Geometry check sheet. Reference: the model listing, model coordinates, mm. A direction names the side the tool comes from. Round coordinates to 2 decimals unless told otherwise and drop trailing zeros. Loops run counter-clockwise (first coordinate to the right, second up) from the corner with the lowest first, then second, coordinate; pieces in that order, holes last. Notation, with made-up numbers: M -17,71 L -12,71 A24 ccw -12,89 Z; hole C 14.5,31 d7. An arc over 180 degrees is marked long. Answer in a Markdown table with one row per item. Add a question column.
```python
from build123d import *

# Parameters (mm, degrees)
BOX035_W               = 60
BOX035_H               = 3
BOX035_DEPTH           = 11
BOX034_W               = 200
BOX034_H               = 30
BOX034_DEPTH           = 20
BOX033_W               = 60
BOX033_H               = 3
BOX033_DEPTH           = 11
BOX025_W               = 3
BOX025_H               = 20
BOX025_DEPTH           = 11
BOX026_W               = 3
BOX026_H               = 20
BOX026_DEPTH           = 11
BOX024_W               = 30
BOX024_H               = 20
BOX024_DEPTH           = 11
BOX023_W               = 20
BOX023_H               = 20
BOX023_DEPTH           = 11
CUT010_PLACEMENT_ANGLE = 180
BOX032_W               = 30
BOX032_H               = 20
BOX032_DEPTH           = 11
BOX031_W               = 20
BOX031_H               = 20
BOX031_DEPTH           = 11
CUT013_PLACEMENT_ANGLE = 180
BOX030_W               = 30
BOX030_H               = 20
BOX030_DEPTH           = 11
BOX029_W               = 20
BOX029_H               = 20
BOX029_DEPTH           = 11
CUT012_PLACEMENT_ANGLE = 180
BOX022_W               = 30
BOX022_H               = 20
BOX022_DEPTH           = 11
BOX021_W               = 20
BOX021_H               = 20
BOX021_DEPTH           = 11
CHAMFER006_SIZE        = 4
BOX018_W               = 178
BOX018_H               = 104
BOX018_DEPTH           = 30
BOX019_W               = 181
BOX019_H               = 121
BOX019_DEPTH           = 5
BOX017_W               = 186
BOX017_H               = 127
BOX017_DEPTH           = 4
FILLET008_R            = 2
FILLET009_R            = 1


with BuildPart() as cube032:
    # Box035 → Box035 (new body)
    with BuildSketch(Plane(origin=(63, 0, 4), x_dir=(1, 0, 0), z_dir=(0, 0, 1))):
        with Locations((30, 1.5)):
            Rectangle(BOX035_W, BOX035_H)
    extrude(amount=BOX035_DEPTH)


with BuildPart() as cube031:
    # Box034 → Box034 (new body)
    with BuildSketch(Plane(origin=(-10, 73, -5), x_dir=(1, 0, 0), z_dir=(0, 0, 1))):
        with Locations((100, 15)):
            Rectangle(BOX034_W, BOX034_H)
    extrude(amount=BOX034_DEPTH)


with BuildPart() as cube030:
    # Box033 → Box033 (new body)
    with BuildSketch(Plane(origin=(63, 112, 4), x_dir=(1, 0, 0), z_dir=(0, 0, 1))):
        with Locations((30, 1.5)):
            Rectangle(BOX033_W, BOX033_H)
    extrude(amount=BOX033_DEPTH)


with BuildPart() as cube022:
    # Box025 → Box025 (new body)
    with BuildSketch(Plane(origin=(0, 50, 4), x_dir=(1, 0, 0), z_dir=(0, 0, 1))):
        with Locations((1.5, 10)):
            Rectangle(BOX025_W, BOX025_H)
    extrude(amount=BOX025_DEPTH)


with BuildPart() as cube023:
    # Box026 → Box026 (new body)
    with BuildSketch(Plane(origin=(183, 50, 4), x_dir=(1, 0, 0), z_dir=(0, 0, 1))):
        with Locations((1.5, 10)):
            Rectangle(BOX026_W, BOX026_H)
    extrude(amount=BOX026_DEPTH)


with BuildPart() as cube021:
    # Box024 → Box024 (new body)
    with BuildSketch(Plane(origin=(3, 3, 0), x_dir=(1, 0, 0), z_dir=(0, 0, 1))):
        with Locations((15, 10)):
            Rectangle(BOX024_W, BOX024_H)
    extrude(amount=BOX024_DEPTH)


with BuildPart() as cut010:
    # Box023 → Box023 (new body)
    with BuildSketch(Plane.XY):
        with Locations((10, 10)):
            Rectangle(BOX023_W, BOX023_H)
    extrude(amount=BOX023_DEPTH)

    # Cut010: cut Cube021
    add(cube021.part, mode=Mode.SUBTRACT)


with BuildPart() as cut010_1:
    # Cut010 placement: moved
    add(cut010.part.moved(Location((186, 0, 15))).rotate(Axis((186, 0, 15), (0, 1, 0)), CUT010_PLACEMENT_ANGLE))


with BuildPart() as cube029:
    # Box032 → Box032 (new body)
    with BuildSketch(Plane(origin=(3, 3, 0), x_dir=(1, 0, 0), z_dir=(0, 0, 1))):
        with Locations((15, 10)):
            Rectangle(BOX032_W, BOX032_H)
    extrude(amount=BOX032_DEPTH)


with BuildPart() as cut013:
    # Box031 → Box031 (new body)
    with BuildSketch(Plane.XY):
        with Locations((10, 10)):
            Rectangle(BOX031_W, BOX031_H)
    extrude(amount=BOX031_DEPTH)

    # Cut013: cut Cube029
    add(cube029.part, mode=Mode.SUBTRACT)


with BuildPart() as cut013_1:
    # Cut013 placement: moved
    add(cut013.part.moved(Location((186, 115, 4))).rotate(Axis((186, 115, 4), (0, 0, 1)), CUT013_PLACEMENT_ANGLE))


with BuildPart() as cube027:
    # Box030 → Box030 (new body)
    with BuildSketch(Plane(origin=(3, 3, 0), x_dir=(1, 0, 0), z_dir=(0, 0, 1))):
        with Locations((15, 10)):
            Rectangle(BOX030_W, BOX030_H)
    extrude(amount=BOX030_DEPTH)


with BuildPart() as cut012:
    # Box029 → Box029 (new body)
    with BuildSketch(Plane.XY):
        with Locations((10, 10)):
            Rectangle(BOX029_W, BOX029_H)
    extrude(amount=BOX029_DEPTH)

    # Cut012: cut Cube027
    add(cube027.part, mode=Mode.SUBTRACT)


with BuildPart() as cut012_1:
    # Cut012 placement: moved
    add(cut012.part.moved(Location((0, 115, 15))).rotate(Axis((0, 115, 15), (1, 0, 0)), CUT012_PLACEMENT_ANGLE))


with BuildPart() as cube019:
    # Box022 → Box022 (new body)
    with BuildSketch(Plane(origin=(3, 3, 0), x_dir=(1, 0, 0), z_dir=(0, 0, 1))):
        with Locations((15, 10)):
            Rectangle(BOX022_W, BOX022_H)
    extrude(amount=BOX022_DEPTH)


with BuildPart() as chamfer006:
    # Box021 → Box021 (new body)
    with BuildSketch(Plane.XY):
        with Locations((10, 10)):
            Rectangle(BOX021_W, BOX021_H)
    extrude(amount=BOX021_DEPTH)

    # Cut009: cut Cube019
    add(cube019.part, mode=Mode.SUBTRACT)


with BuildPart() as chamfer006_1:
    # Cut009 placement: moved
    add(chamfer006.part.moved(Location((0, 0, 4))))

    # Fusion014: union Cube022, Cube023, Cut010, Cut013, Cut012
    add(cube022.part)
    add(cube023.part)
    add(cut010_1.part)
    add(cut013_1.part)
    add(cut012_1.part)

    # Fusion015: union Cube030
    add(cube030.part)

    # Cut014: cut Cube031
    add(cube031.part, mode=Mode.SUBTRACT)

    # Fusion016: union Cube032
    add(cube032.part)

    # Chamfer006
    chamfer006_edges = [chamfer006_1.edges().sort_by_distance(p)[0] for p in [
        (184.5, 20, 15),
        (166, 1.5, 15),
        (63, 113.5, 15),
        (123, 113.5, 15),
        (1.5, 103, 15),
        (20, 113.5, 15),
        (184.5, 50, 15),
        (184.5, 70, 15),
        (184.5, 103, 15),
        (166, 113.5, 15),
        (63, 1.5, 15),
        (123, 1.5, 15),
        (1.5, 50, 15),
        (1.5, 70, 15),
        (1.5, 20, 15),
        (20, 1.5, 15),
    ]]
    chamfer(chamfer006_edges, length=CHAMFER006_SIZE)


with BuildPart() as cutout:
    # Box018 → Box018 (new body)
    with BuildSketch(Plane(origin=(4, 8, -25), x_dir=(1, 0, 0), z_dir=(0, 0, 1))):
        with Locations((89, 52)):
            Rectangle(BOX018_W, BOX018_H)
    extrude(amount=BOX018_DEPTH)


with BuildPart() as cube016:
    # Box019 → Box019 (new body)
    with BuildSketch(Plane(origin=(2.5, 3, -5), x_dir=(1, 0, 0), z_dir=(0, 0, 1))):
        with Locations((90.5, 60.5)):
            Rectangle(BOX019_W, BOX019_H)
    extrude(amount=BOX019_DEPTH)


with BuildPart() as fascia_complete:
    # Box017 → Box017 (new body)
    with BuildSketch(Plane.XY):
        with Locations((93, 63.5)):
            Rectangle(BOX017_W, BOX017_H)
    extrude(amount=BOX017_DEPTH)

    # Fusion007: union Cube016
    add(cube016.part)

    # Cut007: cut Cutout
    add(cutout.part, mode=Mode.SUBTRACT)

    # Fillet008
    fillet008_edges = [fascia_complete.edges().sort_by_distance(p)[0] for p in [
        (183.5, 124, -2.5),
        (2.5, 124, -2.5),
        (2.5, 3, -2.5),
        (183.5, 3, -2.5),
    ]]
    fillet(fillet008_edges, radius=FILLET008_R)

    # Fillet009
    fillet009_edges = [fascia_complete.edges().sort_by_distance(p)[0] for p in [
        (93, 124, -5),
        (3.085786, 123.414214, -5),
        (182.914214, 123.414214, -5),
        (2.5, 63.5, -5),
        (183.5, 63.5, -5),
        (3.085786, 3.585786, -5),
        (182.914214, 3.585786, -5),
        (93, 3, -5),
    ]]
    fillet(fillet009_edges, radius=FILLET009_R)

    # Fusion017: union Chamfer006
    add(chamfer006_1.part)


solid = fascia_complete.part
```
1) Cross-section at C-C, the plane z = 8.75. Count the separate pieces of the cut face and the enclosed holes in it, plus the area to 3 significant figures.
2) Draft check along Y on faces 4 (the flat face through (18, 114, 13)), 5 (the flat face through (92, 3, -2)), 6 (the flat face through (1, 52, 13)). Enter one of: +Y half, -Y half, draft (parallel to the pull), parting line (faces both ways), or undercut.
3) Set-up check for faces 1 (the flat face through (3, 11, 9)), 2 (the flat face through (168, 114, 13)), 3 (the flat face through (92, 124, -2)): record each of +Z, -Z, +X, -X, +Y, -Y from which the full face is reachable in a straight line by a thin tool's end or side.
4) Cross-section at A-A, the plane y = 64. Record the boundary of the cut face in (x, z).
5) Thickness scan on L1, parallel to X at y = 31, z = -2; L2, parallel to Y at x = 64, z = 10.5; L3, parallel to X at y = 10, z = 6.5. Record the ranges inside material, lowest first. Write a range as [from, to].
6) Cross-section at D-D, the plane y = 35.5. Record the boundary of the cut face in (x, z), plus the area to 3 significant figures.
7) Go/stop test with flat-tipped pins: pin 1 (3.5 mm diameter, centred on y = 1, z = 9, fed in from -X); pin 2 (12 mm diameter, centred on x = 13, z = 11.5, fed in from +Y); pin 3 (3 mm diameter, centred on y = 59, z = -2, fed in from +X). Record where each tip stops, or that it passes through.
8) Cross-section at B-B, the plane x = 33. Record the boundary of the cut face in (y, z), plus the area to 3 significant figures.
Worked answers:
| question | item | result |
|---|---|---|
| 1 | separate pieces | 8 |
| 1 | enclosed holes | 0 |
| 1 | area | 876 mm2 |
| 2 | face 4 | draft |
| 2 | face 5 | -Y half |
| 2 | face 6 | undercut |
| 3 | face 1 | +Z |
| 3 | face 2 | +Z, +Y, -Y |
| 3 | face 3 | -Z, +X, -X, +Y |
| 4 | outline | M 0,0 L 2.5,0 L 2.5,-4 A1 ccw 3.5,-5 L 4,-5 L 4,4 L 3,4 L 3,15 L 0,15 Z; M 182,-5 L 182.5,-5 A1 ccw 183.5,-4 L 183.5,0 L 186,0 L 186,15 L 183,15 L 183,4 L 182,4 Z |
| 5 | L1 | x = [2.5, 4], [182, 183.5] |
| 5 | L2 | y = [0, 3], [112, 115] |
| 5 | L3 | x = [0, 3], [183, 186] |
| 6 | outline | M 0,0 L 2.5,0 L 2.5,-4 A1 ccw 3.5,-5 L 4,-5 L 4,4 L 0,4 Z; M 182,-5 L 182.5,-5 A1 ccw 183.5,-4 L 183.5,0 L 186,0 L 186,4 L 182,4 Z |
| 6 | area | 46.6 mm2 |
| 7 | pin 1 | stops at x = 0 |
| 7 | pin 2 | stops at y = 115 |
| 7 | pin 3 | stops at x = 183.5 |
| 8 | outline | M 0,0 L 3,0 L 3,-4 A1 ccw 4,-5 L 8,-5 L 8,4 L 0,4 Z; M 112,-5 L 123,-5 A1 ccw 124,-4 L 124,0 L 127,0 L 127,4 L 112,4 Z |
| 8 | area | 177 mm2 |
